The model under review builds one solid part; all positions refer to its coordinate system, in mm. Face numbers are marked on the shaded views. A direction names the side the tool comes from. Coordinates: 2 decimals unless noted, no trailing zeros. Order: outer loops, then holes, each group sorted by start corner. A loop starts at its lowest first (then second) coordinate and runs counter-clockwise, first axis right, second up. Notation, with made-up numbers: (-23.75, 68) -> (22.25, 68) arc R16 ccw to (22.25, 87) -> close; hole circle Ø1 at (85.25, -20.75). An arc over 180 degrees is marked (long way). Use CSV: the item, a comma, the result in double quotes. Start each with the question number.
```python
from build123d import *

# Parameters (mm, degrees)
SKETCH1_R           = 3.175
BOSS_EXTRUDE2_DEPTH = 90
SKETCH1_4_R         = 5
SKETCH1_4_R_2       = 3.175
BOSS_EXTRUDE3_DEPTH = 60


with BuildPart() as part:
    # Sketch1 → Boss-Extrude2 (new, symmetric)
    with BuildSketch(Plane(origin=(0, 0, 0), x_dir=(1, 0, 0), z_dir=(0, 1, 0))):
        Circle(SKETCH1_R)
    extrude(amount=BOSS_EXTRUDE2_DEPTH, both=True)

    # Sketch1<4> → Boss-Extrude3 (add, symmetric)
    with BuildSketch(Plane(origin=(0, 0, 0), x_dir=(1, 0, 0), z_dir=(0, 1, 0))):
        Circle(SKETCH1_4_R)
        Circle(SKETCH1_4_R_2, mode=Mode.SUBTRACT)
    extrude(amount=BOSS_EXTRUDE3_DEPTH, both=True)


solid = part.part
```
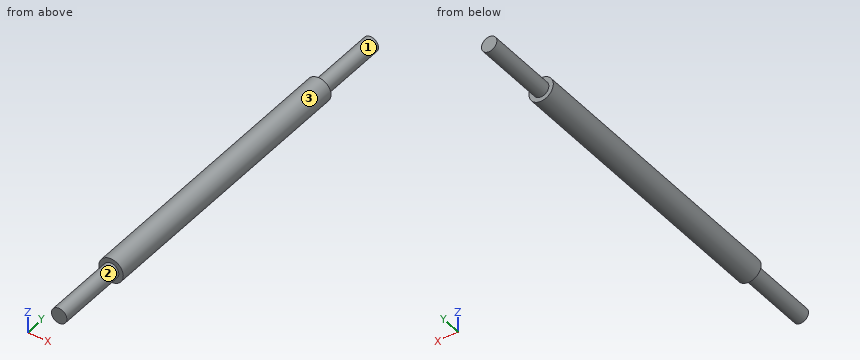
Q1. To check wall thickness, follow probe 1 along X at (y, z) = (-22, 0.25); probe 2 along Z at (x, y) = (-0.5, -3); probe 3 along Y at (x, z) = (-3.5, 0.25). State the ranges of each line that lie inside material, in increasing order.
Q2. For the marked faces 1, 2 and 3, list the 3-axis set-ups (+Z, -Z, +X, -X, +Y, -Y) from which the entire face can be reached by the end or side of a thin tool; tool diameter is ignored.
Q3. Clearance check with flat-ended pins moving along their axes: pin 1 Ø6 at (y, z) = (35.5, 2) entering from +X; pin 2 Ø6 at (y, z) = (70.5, 1) entering from -X (3 decimals); pin 3 Ø1.5 at (x, y) = (-2, 34) entering from -Z; pin 4 Ø1 at (x, z) = (3.5, -1.5) entering from +Y. State where each tip first meets the part, or that it passes through.
Q4. Add section A-A, the plane z = 0. State the section outline as (x, y) points (3 decimals), then the cut area to 3 significant figures.
Q5. Add section B-B, the plane x = 0. State the section outline as (y, z) points (3 decimals), then the cut area to 3 significant figures.
Q6. Add section C-C, the plane y = 26.5. State the section outline as (x, z) points.
Q7. Add section D-D, the plane y = 70.5. State the section outline as (x, z) points (3 decimals).
Answer block:
1,probe 1,"x = -4.99 to 4.99"
1,probe 2,"z = -4.97 to 4.97"
1,probe 3,"y = -60 to 60"
2,face 1,"+Y"
2,face 2,"-Y"
2,face 3,"+Y, -Y"
3,pin 1,"stops at x = 5"
3,pin 2,"stops at x = -3.175"
3,pin 3,"stops at z = -4.84"
3,pin 4,"stops at y = 60"
4,outline,"(-5, -60) -> (-3.175, -60) -> (-3.175, -90) -> (3.175, -90) -> (3.175, -60) -> (5, -60) -> (5, 60) -> (3.175, 60) -> (3.175, 90) -> (-3.175, 90) -> (-3.175, 60) -> (-5, 60) -> close"
4,area,"1,580 mm²"
5,outline,"(-90, -3.175) -> (-60, -3.175) -> (-60, -5) -> (60, -5) -> (60, -3.175) -> (90, -3.175) -> (90, 3.175) -> (60, 3.175) -> (60, 5) -> (-60, 5) -> (-60, 3.175) -> (-90, 3.175) -> close"
5,area,"1,580 mm²"
6,outline,"circle Ø10 at (0, 0)"
7,outline,"circle Ø6.35 at (0, 0)"
